Geometry check sheet. Reference: the model listing, model coordinates, mm. Face numbers are marked on the shaded views. Give positions to 0.01 mm unless a question says otherwise; leave off trailing zeros. Loops run counter-clockwise (first coordinate to the right, second up) from the corner with the lowest first, then second, coordinate; pieces in that order, holes last.
1. Cross-section at B-B, the plane y = 10.25. Record the cut outline in (x, z) (3 decimals).
2. Cross-section at D-D, the plane y = 3. Record the cut outline in (x, z), plus the area to 3 significant figures.
3. Release check for a two-part mould opening along X. For the marked faces 1 and 2 record: +X half, -X half, draft (parallel to the pull), parting line (faces both ways), or undercut.
4. Go/stop test with flat-tipped pins: pin 1 Ø1 at (x, y) = (-5.5, 7.5) entering from +Z; pin 2 Ø3 at (y, z) = (8.5, -12) entering from +X; pin 3 Ø3 at (x, z) = (11, -4.5) entering from -Y; pin 4 Ø2.5 at (x, z) = (-3.5, 16) entering from +Y. Record where each tip stops, or that it passes through.
5. Material ranges on L1, parallel to X at y = 4, z = -12; L2, parallel to X at y = 14.5, z = -7.5 (3 decimals); L3, parallel to Z at x = -11.5, y = 1.5, recorded low to high.
6. Cross-section at A-A, the plane x = 0. Record the cut outline in (y, z), plus the area to 3 significant figures.
7. Cross-section at C-C, the plane z = 13.5. Record the cut outline in (x, y) (3 decimals), plus the area to 3 significant figures.
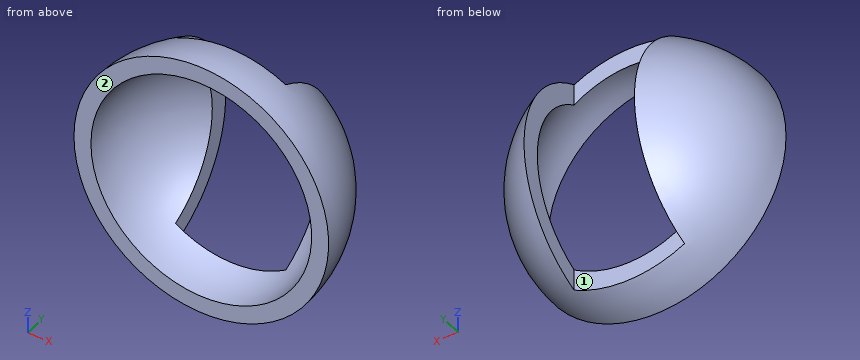
from build123d import *

# Parameters (mm, degrees)
SKETCH2_W          = 16.51
SKETCH2_H          = 16.418842622
CUT_EXTRUDE1_DEPTH = 63.5


with BuildPart() as part:
    # Sketch1 → Revolve1 (revolve)
    with BuildSketch(Plane.XY, mode=Mode.PRIVATE) as revolve1_sk:
        with BuildLine():
            Line((19.05, 0), (16.51, 0))
            ThreePointArc((16.51, 0), (11.674332957, 11.674332957), (0, 16.51))
            Line((0, 16.51), (0, 19.05))
            ThreePointArc((0, 19.05), (13.470384182, 13.470384182), (19.05, 0))
        make_face()
    revolve(revolve1_sk.sketch.rotate(Axis((0, 19.05, 0), (0, -1, 0)), 180), axis=Axis((0, 19.05, 0), (0, -1, 0)))

    # Sketch2 → Cut-Extrude1 (cut, symmetric)
    with BuildSketch(Plane.XY):
        with Locations((0, 14.559421311)):
            Rectangle(SKETCH2_W, SKETCH2_H)
    extrude(amount=CUT_EXTRUDE1_DEPTH, both=True, mode=Mode.SUBTRACT)


solid = part.part
Result:
1. outline: (-8.255, -13.773) - (-8.255, -9.969) arc R12.943 cw to (-8.255, 9.969) - (-8.255, 13.773) arc R16.057 ccw to start; (8.255, -13.773) arc R16.057 ccw to (8.255, 13.773) - (8.255, 9.969) arc R12.943 cw to (8.255, -9.969) - close
2. outline: circle Ø37.62 at (0, 0); hole circle Ø32.47 at (0, 0)
2. area: 284 mm2
3. face 1: undercut
3. face 2: draft
4. pin 1: passes through
4. pin 2: stops at x = 13.73
4. pin 3: stops at y = 9.67
4. pin 4: stops at y = 6.35
5. L1: x = -14.24 to -10.61, 10.61 to 14.24
5. L2: x = -9.818 to -8.255, 8.255 to 9.818
5. L3: z = -15.11 to -11.75, 11.75 to 15.11
6. outline: (0, -19.05) arc R19.05 ccw to (6.35, -17.96) - (6.35, -15.24) arc R16.51 cw to (0, -16.51) - close; (0, 16.51) arc R16.51 cw to (6.35, 15.24) - (6.35, 17.96) arc R19.05 ccw to (0, 19.05) - close
6. area: 33.0 mm2
7. outline: (-13.441, 0) - (-9.504, 0) arc R9.504 cw to (-7.072, 6.35) - (-8.255, 6.35) - (-8.255, 10.607) arc R13.441 ccw to start; (7.072, 6.35) arc R9.504 cw to (9.504, 0) - (13.441, 0) arc R13.441 ccw to (8.255, 10.607) - (8.255, 6.35) - close
7. area: 70.6 mm2
